```python
from build123d import *

# Parameters (mm, degrees)
SKETCH1_R               = 16
SKETCH1_R_2             = 1.75
SKETCH1_R_3             = 8
BOSS_EXTRUDE1_DEPTH     = 3
SKETCH1_3_R             = 8
SKETCH1_3_R_2           = 3.8
BOSS_EXTRUDE2_DEPTH     = 13
SKETCH2_R               = 1.944334414
CUT_EXTRUDE1_DEPTH      = 17
CUT_EXTRUDE1_DEPTH_BACK = 17


with BuildPart() as part:
    # Sketch1 → Boss-Extrude1 (new body)
    with BuildSketch(Plane(origin=(0, 0, 0), x_dir=(1, 0, 0), z_dir=(0, 1, 0))):
        Circle(SKETCH1_R)
        with Locations((-11.75, 0)):
            Circle(SKETCH1_R_2, mode=Mode.SUBTRACT)
        with Locations((0, -11.75)):
            Circle(SKETCH1_R_2, mode=Mode.SUBTRACT)
        with Locations((11.75, 0)):
            Circle(SKETCH1_R_2, mode=Mode.SUBTRACT)
        with Locations((0, 11.75)):
            Circle(SKETCH1_R_2, mode=Mode.SUBTRACT)
        Circle(SKETCH1_R_3, mode=Mode.SUBTRACT)
    extrude(amount=BOSS_EXTRUDE1_DEPTH)

    # Sketch1<3> → Boss-Extrude2 (add)
    with BuildSketch(Plane(origin=(0, 0, 0), x_dir=(1, 0, 0), z_dir=(0, 1, 0))):
        Circle(SKETCH1_3_R)
        Circle(SKETCH1_3_R_2, mode=Mode.SUBTRACT)
    extrude(amount=BOSS_EXTRUDE2_DEPTH)

    # Sketch2 → Cut-Extrude1 (cut, two sides)
    with BuildSketch(Plane.XY) as cut_extrude1_sk:
        with Locations((0, 8)):
            Circle(SKETCH2_R)
    extrude(amount=CUT_EXTRUDE1_DEPTH, mode=Mode.SUBTRACT)
    extrude(cut_extrude1_sk.sketch, amount=-CUT_EXTRUDE1_DEPTH_BACK, mode=Mode.SUBTRACT)


solid = part.part
```
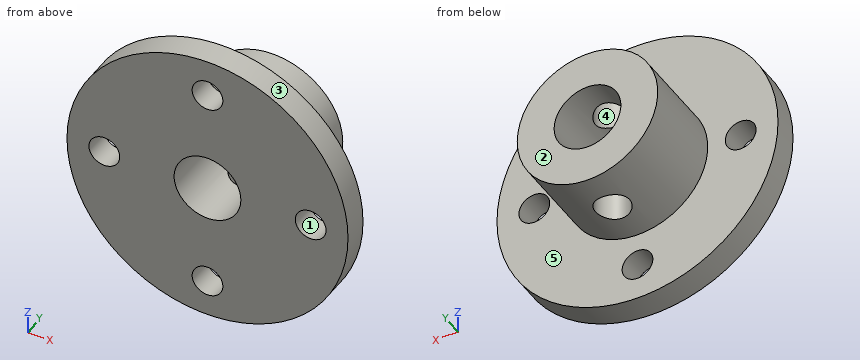
Input: part model. Units: mm. Frame: model coordinates. Face numbers are marked on the shaded views. A direction names the side the tool comes from. Round coordinates to 2 decimals unless told otherwise and drop trailing zeros. Write each loop counter-clockwise with the first axis right and the second up, starting at its lowest first coordinate (ties: lowest second). Pieces come first, ordered by that corner, then holes. Notation, with made-up numbers: M 13.5,47.25 L 42.5,47.25 A24 cw 42.5,83.25 Z; hole C -11.75,-32.75 d4. An arc over 180 degrees is marked long. Write each question's results on one line, items separated by ' | '.
Q1. Section query B-B (x = 12). Return loops of the section in (y, z).
Results:
outline: M 0,-10.58 L 3,-10.58 L 3,-1.73 L 0,-1.73 Z; M 0,1.73 L 3,1.73 L 3,10.58 L 0,10.58 Z
Q2. Section query A-A (y = 8.5). Return loops of the section in (x, z), and give its area (3 significant figures).
Results:
outline: M -1.88,-7.78 L -1.88,-3.3 A3.8 cw -1.88,3.3 L -1.88,7.78 A8 ccw Z; M 1.88,-7.78 A8 ccw 1.88,7.78 L 1.88,3.3 A3.8 cw 1.88,-3.3 Z | area: 123 mm^2
Q3. Access query for the marked faces 4 and 5. Directions: +Z, -Z, +X, -X, +Y, -Y. A direction counts if a zero-diameter tool reaches every point of the face in a straight line with its end or side. Return the directions, or none.
Results:
face 4: +Z, -Z | face 5: +Y
Q4. Pin query (flat end, axial travel): P1, Ø4, axis at x = -11.75, z = 0, coming from the +Y side; P2, Ø4.5, axis at x = 0, z = 0, coming from the -Y side; P3, Ø4, axis at y = 3, z = -7, coming from the +X side; P4, Ø1.5, axis at x = -6.5, y = 10.5, coming from the +Z side. Return the tip coordinate at first contact, or that it passes through.
Results:
P1: stops at y = 3 | P2: passes through | P3: stops at x = 15.2 | P4: stops at z = 5.56
Q5. Draft query along X for the marked faces 1, 2 and 3. Return one class per face: released by +X, released by -X, zero draft, split by the parting line, or undercut.
Results:
face 1: undercut | face 2: zero draft | face 3: split by the parting line
Q6. Line query: line 1 along X through (y, z) = (1.3, 0); line 2 along Y through (x, z) = (12, 3). Output: solid intervals per line, ascending.
Results:
line 1: x = -16 to -13.5, -10 to -3.8, 3.8 to 10, 13.5 to 16 | line 2: y = 0 to 3
Q7. Section query C-C (y = 1). Return loops of the section in (x, z), and give its area (3 significant figures).
Results:
outline: C 0,0 d32; hole C -11.75,0 d3.5; hole C 0,0 d7.6; hole C 0,-11.75 d3.5; hole C 0,11.75 d3.5; hole C 11.75,0 d3.5 | area: 720 mm^2
Q8. Section query D-D (y = 12). Return loops of the section in (x, z), and give its area (3 significant figures).
Results:
outline: C 0,0 d16; hole C 0,0 d7.6 | area: 156 mm^2
